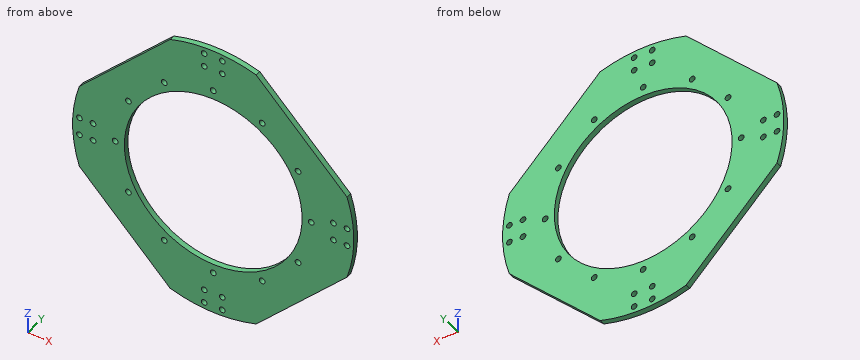
```python
from build123d import *

# Parameters (mm, degrees)
SKETCH_1_R          = 77.5
SKETCH_1_R_2        = 49
SKETCH_1_R_3        = 1.6
SKETCH_1_R_4        = 1.575
EXTRUDE_1_DEPTH     = 3
CUT_EXTRUDE_1_DEPTH = 10


with BuildPart() as part:
    # 草图1 → 凸台-拉伸1 (new body)
    with BuildSketch(Plane(origin=(0, 0, 0), x_dir=(1, 0, 0), z_dir=(0, 1, 0))):
        with Locations(Location((0, 0, 0), (0, 0, 270))):
            Circle(SKETCH_1_R)
        with Locations(Location((0, 0, 0), (0, 0, 270))):
            Circle(SKETCH_1_R_2, mode=Mode.SUBTRACT)
        with Locations(Location((0, 54, 0), (0, 0, 270))):
            Circle(SKETCH_1_R_3, mode=Mode.SUBTRACT)
        with Locations(Location((27, 46.765371804, 0), (0, 0, 270))):
            Circle(SKETCH_1_R_3, mode=Mode.SUBTRACT)
        with Locations(Location((46.765371804, 27, 0), (0, 0, 270))):
            Circle(SKETCH_1_R_3, mode=Mode.SUBTRACT)
        with Locations(Location((54, 0, 0), (0, 0, 270))):
            Circle(SKETCH_1_R_3, mode=Mode.SUBTRACT)
        with Locations(Location((46.765371804, -27, 0), (0, 0, 270))):
            Circle(SKETCH_1_R_3, mode=Mode.SUBTRACT)
        with Locations(Location((27, -46.765371804, 0), (0, 0, 270))):
            Circle(SKETCH_1_R_3, mode=Mode.SUBTRACT)
        with Locations(Location((0, -54, 0), (0, 0, 270))):
            Circle(SKETCH_1_R_3, mode=Mode.SUBTRACT)
        with Locations(Location((-27, -46.765371804, 0), (0, 0, 270))):
            Circle(SKETCH_1_R_3, mode=Mode.SUBTRACT)
        with Locations(Location((-46.765371804, -27, 0), (0, 0, 270))):
            Circle(SKETCH_1_R_3, mode=Mode.SUBTRACT)
        with Locations(Location((-54, 0, 0), (0, 0, 270))):
            Circle(SKETCH_1_R_3, mode=Mode.SUBTRACT)
        with Locations(Location((-46.765371804, 27, 0), (0, 0, 270))):
            Circle(SKETCH_1_R_3, mode=Mode.SUBTRACT)
        with Locations(Location((-27, 46.765371804, 0), (0, 0, 270))):
            Circle(SKETCH_1_R_3, mode=Mode.SUBTRACT)
        with Locations(Location((-73.75, 5, 0), (0, 0, 270))):
            Circle(SKETCH_1_R_4, mode=Mode.SUBTRACT)
        with Locations(Location((-66.25, 5, 0), (0, 0, 90))):
            Circle(SKETCH_1_R_4, mode=Mode.SUBTRACT)
        with Locations(Location((-66.25, -5, 0), (0, 0, 270))):
            Circle(SKETCH_1_R_4, mode=Mode.SUBTRACT)
        with Locations(Location((-73.75, -5, 0), (0, 0, 90))):
            Circle(SKETCH_1_R_4, mode=Mode.SUBTRACT)
        with Locations(Location((5, 73.75, 0), (0, 0, 270))):
            Circle(SKETCH_1_R_4, mode=Mode.SUBTRACT)
        with Locations(Location((5, 66.25, 0), (0, 0, 90))):
            Circle(SKETCH_1_R_4, mode=Mode.SUBTRACT)
        with Locations(Location((-5, 66.25, 0), (0, 0, 270))):
            Circle(SKETCH_1_R_4, mode=Mode.SUBTRACT)
        with Locations(Location((-5, 73.75, 0), (0, 0, 90))):
            Circle(SKETCH_1_R_4, mode=Mode.SUBTRACT)
        with Locations(Location((73.75, -5, 0), (0, 0, 270))):
            Circle(SKETCH_1_R_4, mode=Mode.SUBTRACT)
        with Locations(Location((66.25, -5, 0), (0, 0, 90))):
            Circle(SKETCH_1_R_4, mode=Mode.SUBTRACT)
        with Locations(Location((66.25, 5, 0), (0, 0, 270))):
            Circle(SKETCH_1_R_4, mode=Mode.SUBTRACT)
        with Locations(Location((73.75, 5, 0), (0, 0, 90))):
            Circle(SKETCH_1_R_4, mode=Mode.SUBTRACT)
        with Locations(Location((-5, -73.75, 0), (0, 0, 270))):
            Circle(SKETCH_1_R_4, mode=Mode.SUBTRACT)
        with Locations(Location((-5, -66.25, 0), (0, 0, 90))):
            Circle(SKETCH_1_R_4, mode=Mode.SUBTRACT)
        with Locations(Location((5, -66.25, 0), (0, 0, 270))):
            Circle(SKETCH_1_R_4, mode=Mode.SUBTRACT)
        with Locations(Location((5, -73.75, 0), (0, 0, 90))):
            Circle(SKETCH_1_R_4, mode=Mode.SUBTRACT)
    extrude(amount=EXTRUDE_1_DEPTH)

    # 草图2 → 切除-拉伸1 (cut)
    with BuildSketch(Plane.XZ):
        with BuildLine():
            ThreePointArc((73.781230493, 23.718769507), (54.800775542, 54.800775542), (23.718769507, 73.781230493))
            Line((23.718769507, 73.781230493), (73.781230493, 23.718769507))
        make_face()
        with BuildLine():
            Line((73.781230493, -23.718769507), (23.718769507, -73.781230493))
            ThreePointArc((23.718769507, -73.781230493), (54.800775542, -54.800775542), (73.781230493, -23.718769507))
        make_face()
        with BuildLine():
            Line((-73.781230493, 23.718769507), (-23.718769507, 73.781230493))
            ThreePointArc((-23.718769507, 73.781230493), (-54.800775542, 54.800775542), (-73.781230493, 23.718769507))
        make_face()
        with BuildLine():
            Line((-23.718769507, -73.781230493), (-73.781230493, -23.718769507))
            ThreePointArc((-73.781230493, -23.718769507), (-54.800775542, -54.800775542), (-23.718769507, -73.781230493))
        make_face()
    extrude(amount=-CUT_EXTRUDE_1_DEPTH, mode=Mode.SUBTRACT)


solid = part.part
```
Design review of the part built by this model. Coordinates are the model's own, in mm. Coordinates: 2 decimals unless noted, no trailing zeros. Order: outer loops, then holes, each group sorted by start corner. A loop starts at its lowest first (then second) coordinate and runs counter-clockwise, first axis right, second up. Notation, with made-up numbers: M 15,42 L 63,42 A22 ccw 63,56 Z; hole C 5.5,54.25 d5. An arc over 180 degrees is marked long. Answer as a JSON object with one key per item and string values. Group by question number.
1) Add section A-A, the plane z = 42. Write out the cut boundary in (x, y).
2) For pin 1 (1 mm diameter, centred on y = 1.5, z = 37, fed in from -X), flat-tipped, find the tip position at first contact; note if it passes through.
3) Add section B-B, the plane z = -57.5. Write out the cut boundary in (x, y), then the cut area to 3 significant figures.
4) Wall thickness on L1, parallel to Z at x = -73.75, y = 2.2 (3 decimals); L2, parallel to Z at x = 66.25, y = 2 (3 decimals); L3, parallel to X at y = 1.4, z = 27: over which ranges is each line inside the solid? List them lowest first.
5) Add section C-C, the plane y = 0.8. Count the separate pieces of the cut face and the enclosed holes in it, then the cut area to 3 significant figures.
Computed values:
{
 "1": {"outline": "M -55.5,0 L -25.24,0 L -25.24,3 L -55.5,3 Z; M 25.24,0 L 55.5,0 L 55.5,3 L 25.24,3 Z"},
 "2": {"pin 1": "stops at x = -61"},
 "3": {"outline": "M -40,0 L 40,0 L 40,3 L -40,3 Z", "area": "240 mm^2"},
 "4": {"L1": "z = -23.75 to -6.575, -3.425 to 3.425, 6.575 to 23.75", "L2": "z = -31.25 to -6.575, -3.425 to 3.425, 6.575 to 31.25", "L3": "x = -70.5 to -48.37, -45.17 to -40.89, 40.89 to 45.17, 48.37 to 70.5"},
 "5": {"separate pieces": "1", "enclosed holes": "29", "area": "9,470 mm^2"}
}
